```python
from build123d import *

# Parameters (mm, degrees)
BOSS_EXTRUDE1_DEPTH     = 70
CUT_EXTRUDE1_DEPTH      = 309.220700148
CUT_EXTRUDE1_DEPTH_BACK = 3
SKETCH3_W               = 300
SKETCH3_H               = 3
CUT_EXTRUDE2_DEPTH      = 2


with BuildPart() as part:
    # Sketch1 → Boss-Extrude1 (new body)
    with BuildSketch(Plane(origin=(0, 0, 0), x_dir=(1, 0, 0), z_dir=(0, 1, 0))):
        Polygon((0, 10), (10, 0), (290, 0), (300, 10), align=None)
    extrude(amount=BOSS_EXTRUDE1_DEPTH)

    # Sketch2 → Cut-Extrude1 (cut, two sides: drawn at the far end of the back side and taken through both)
    with BuildSketch(Plane(origin=(0, 70, 0), x_dir=(1, 0, 0), z_dir=(0, 1, 0)).offset(-CUT_EXTRUDE1_DEPTH_BACK)):
        Polygon((295, 5), (5, 5), (10, 0), (290, 0), align=None)
    extrude(amount=CUT_EXTRUDE1_DEPTH + CUT_EXTRUDE1_DEPTH_BACK, mode=Mode.SUBTRACT)

    # Sketch3 → Cut-Extrude2 (cut)
    with BuildSketch(Plane.XY):
        with Locations((150, 8.5)):
            Rectangle(SKETCH3_W, SKETCH3_H)
    extrude(amount=-CUT_EXTRUDE2_DEPTH, mode=Mode.SUBTRACT)


solid = part.part
```
Could you check a few things on this model? Use its own coordinates, in mm. A direction names the side the tool comes from. Give positions to 0.01 mm unless a question says otherwise; leave off trailing zeros. Order: outer loops, then holes, each group sorted by start corner. A loop starts at its lowest first (then second) coordinate and runs counter-clockwise, first axis right, second up.
Q1. I'm going to push flat-ended pins straight in: P1, Ø0.6, axis at x = 90, z = -0.5, coming from the -Y side; P2, Ø4, axis at x = 128, z = -2.5, coming from the +Y side; P3, Ø1.5, axis at x = 109, y = 68.5, coming from the +Z side. Where does each tip first touch, or does it pass through?
Q2. Suppose I cut it at A-A, the plane x = 98.5. Write out the boundary of the cut face in (y, z).
Q3. If I drill on line 1 along Y through (x, z) = (59.5, -4.75); line 2 along Y through (x, z) = (58, -1.75); line 3 along X through (y, z) = (64, -5), over which ranges is the centre line in solid material (lowest first)?
Q4. Suppose I cut it at B-B, the plane y = 42.5. Write out the boundary of the cut face in (x, z), and give its area (3 significant figures).
Q5. For faces 1 (the flat face through (148, 67, -3)), 2 (the flat face through (148, 0, -5)), which set-ups out of +Z, -Z, +X, -X, +Y, -Y let a thin tool reach every point of the face, with its end or its side?
Solution:
1. P1: stops at y = 0
1. P2: stops at y = 67
1. P3: stops at z = -5
2. outline: (0, -10) - (70, -10) - (70, -5) - (67, -5) - (67, 0) - (10, 0) - (10, -2) - (7, -2) - (7, 0) - (0, 0) - close
3. line 1: y = 0 to 67
3. line 2: y = 0 to 7, 10 to 67
3. line 3: x = 5 to 295
4. outline: (0, -10) - (300, -10) - (290, 0) - (10, 0) - close
4. area: 2,900 mm2
5. face 1: +Z, +X, -X, +Y
5. face 2: +Z, -Z, +X, -X, -Y
